Source: three-view drawing plus pictorial views. Frame: mm from the lowest corner of the part. A direction names the side the tool comes from. Give positions to 0.01 mm unless a question says otherwise; leave off trailing zeros. Order: outer loops, then holes, each group sorted by start corner. A loop starts at its lowest first (then second) coordinate and runs counter-clockwise, first axis right, second up.
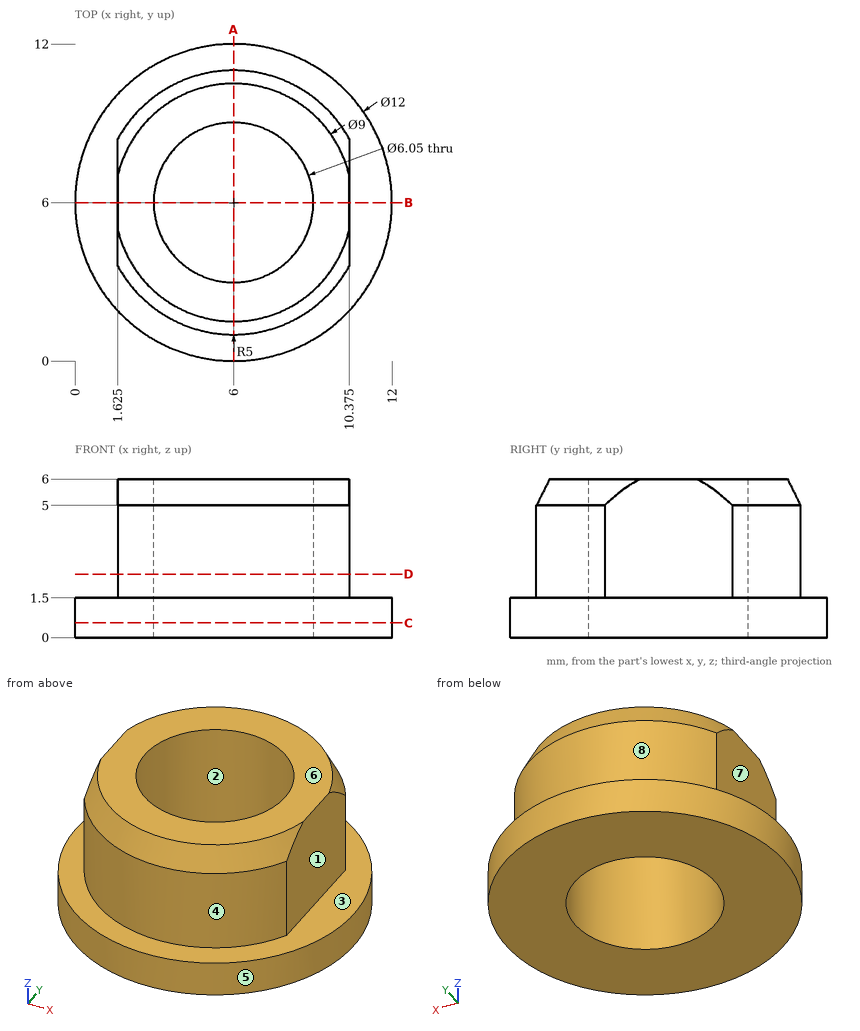
1) Pull-direction query (X, two-part tool) for the marked faces 1, 2 and 3; classes: +X half, -X half, draft (parallel to the pull), parting line (faces both ways), or undercut.
Checks:
face 1: +X half
face 2: undercut
face 3: draft
2) Section query D-D on z = 2.4. Output: boundary loops of the cut face in (x, y) (3 decimals).
Checks:
outline: (1.625, 3.579) arc R5 ccw to (10.375, 3.579) - (10.375, 8.421) arc R5 ccw to (1.625, 8.421) - close; hole circle Ø6.05 at (6, 6)
3) Section query A-A on x = 6. Output: boundary loops of the cut face in (y, z) (3 decimals), and give its area (3 significant figures).
Checks:
outline: (0, 0) - (2.975, 0) - (2.975, 6) - (1.5, 6) - (1, 5) - (1, 1.5) - (0, 1.5) - close; (9.025, 0) - (12, 0) - (12, 1.5) - (11, 1.5) - (11, 5) - (10.5, 6) - (9.025, 6) - close
area: 26.2 mm2
4) First-contact query: pin 1 Ø7 at (x, y) = (6, 6) entering from +Z; pin 2 Ø3 at (y, z) = (2.5, 5) entering from +X (3 decimals); pin 3 Ø2 at (y, z) = (3, 5) entering from -X (3 decimals). Flat tips, straight axial feed; report the tip coordinate or a pass-through.
Checks:
pin 1: stops at z = 6
pin 2: stops at x = 10.375
pin 3: stops at x = 1.625
5) Section query B-B on y = 6. Output: boundary loops of the cut face in (x, z) (3 decimals), and give its area (3 significant figures).
Checks:
outline: (0, 0) - (2.975, 0) - (2.975, 6) - (1.625, 6) - (1.625, 1.5) - (0, 1.5) - close; (9.025, 0) - (12, 0) - (12, 1.5) - (10.375, 1.5) - (10.375, 6) - (9.025, 6) - close
area: 21.1 mm2
6) Reachability of the marked faces 4, 5, 6, 7 and 8 from +Z, -Z, +X, -X, +Y, -Y: full face, straight path, thin tool, end or side. Return the list, or none.
Checks:
face 4: +Z, -Y
face 5: +Z, -Z
face 6: +Z, +X, -X, +Y, -Y
face 7: +Z, -X, +Y, -Y
face 8: +Z, +Y
7) Ray query, L1, parallel to Y at x = 6, z = 2 (3 decimals); L2, parallel to Y at x = 6, z = 1.35 (3 decimals); L3, parallel to Z at x = 9.5, y = 10. Return the intervals inside material, ascending.
Checks:
L1: y = 1 to 2.975, 9.025 to 11
L2: y = 0 to 2.975, 9.025 to 12
L3: z = 0 to 1.5
8) Section query C-C on z = 0.55. Output: boundary loops of the cut face in (x, y) (3 decimals).
Checks:
outline: circle Ø12 at (6, 6); hole circle Ø6.05 at (6, 6)
